Geometry: final body of the model. Coordinates: model frame, mm. Face numbers are marked on the shaded views. A direction names the side the tool comes from. Give positions to 0.01 mm unless a question says otherwise; leave off trailing zeros. Order: outer loops, then holes, each group sorted by start corner. A loop starts at its lowest first (then second) coordinate and runs counter-clockwise, first axis right, second up. Notation, with made-up numbers: (-37, 82) -> (-26, 82) arc R17 ccw to (-26, 96) -> close; hole circle Ø4 at (76, 22). An arc over 180 degrees is marked (long way). One line per item, written item: value. Start each with the question number.
```python
from build123d import *

# Parameters (mm, degrees)
BOSS_EXTRUDE1_DEPTH     = 7.5
CUT_EXTRUDE1_REACH      = 84.651
SKETCH2_R               = 5
CUT_EXTRUDE2_REACH      = 89.839
CUT_EXTRUDE2_END_RADIUS = 39.885527085
SKETCH3_R               = 5


with BuildPart() as part:
    # Sketch1 → Boss-Extrude1 (new, symmetric)
    with BuildSketch(Plane(origin=(0, 0, 0), x_dir=(1, 0, 0), z_dir=(0, 1, 0))):
        with BuildLine():
            Line((-17.171350292, -36), (17.171350292, -36))
            ThreePointArc((17.171350292, -36), (39.885527085, 0), (17.171350292, 36))
            Line((17.171350292, 36), (-17.171350292, 36))
            ThreePointArc((-17.171350292, 36), (-39.885527085, 0), (-17.171350292, -36))
        make_face()
        with BuildLine():
            Line((-16, 31), (16, 31))
            ThreePointArc((16, 31), (34.885527085, 0), (16, -31))
            Line((16, -31), (-16, -31))
            ThreePointArc((-16, -31), (-34.885527085, 0), (-16, 31))
        make_face(mode=Mode.SUBTRACT)
    extrude(amount=BOSS_EXTRUDE1_DEPTH, both=True)

    # Cut-Extrude1: up to this face of the body (flat: up to its plane)
    cut_extrude1_end = Plane(part.part.faces().sort_by_distance((0, 0, -36))[0])
    # Sketch2 → Cut-Extrude1 (cut, up to the picked face)
    with BuildSketch(Plane.XY.offset(36), mode=Mode.PRIVATE) as cut_extrude1_sk1:
        with Locations((0, -0.5)):
            Circle(SKETCH2_R)
    cut_extrude1_tool1 = split(extrude(cut_extrude1_sk1.sketch, amount=-CUT_EXTRUDE1_REACH, mode=Mode.PRIVATE), bisect_by=cut_extrude1_end, keep=Keep.BOTH, mode=Mode.PRIVATE)
    add(cut_extrude1_tool1.solids().sort_by(Axis((0, -0.5, 36), (0, 0, -1)))[0], mode=Mode.SUBTRACT)

    # Cut-Extrude2: up to this cylinder (the profile starts inside it)
    cut_extrude2_end = Plane(origin=(0, 0, 0), z_dir=(0, -1, 0)) * Cylinder(CUT_EXTRUDE2_END_RADIUS, 260.44905417, mode=Mode.PRIVATE)
    # Sketch3 → Cut-Extrude2 (cut, up to the surface)
    with BuildSketch(Plane.ZY.offset(39.885527085), mode=Mode.PRIVATE) as cut_extrude2_sk1:
        Circle(SKETCH3_R)
    cut_extrude2_tool1 = extrude(cut_extrude2_sk1.sketch, amount=-CUT_EXTRUDE2_REACH, mode=Mode.PRIVATE) & cut_extrude2_end
    add(cut_extrude2_tool1.solids().sort_by_distance((-39.885527, 0, 0))[0], mode=Mode.SUBTRACT)


solid = part.part
```
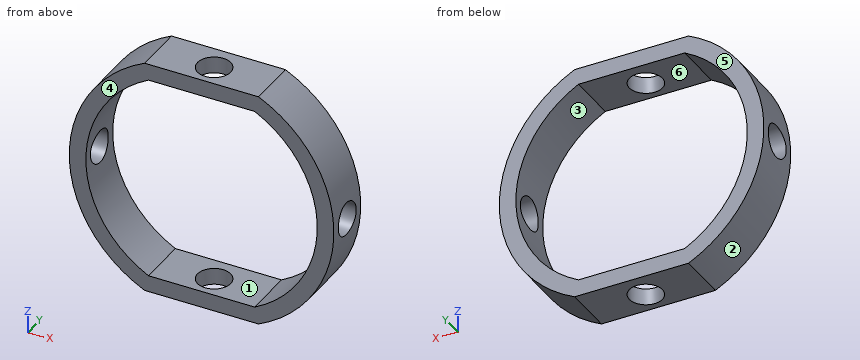
1. Cut plane C-C, the plane y = 1. Return loops of the section in (x, z), then the cut area to 3 significant figures.
2. Pin query (flat end, axial travel): P1, Ø5, axis at x = -22, y = 4, coming from the -Z side; P2, Ø8, axis at y = -6, z = -13, coming from the -X side; P3, Ø6, axis at y = 5, z = 23, coming from the -X side. Return the tip coordinate at first contact, or that it passes through.
3. Cut plane A-A, the plane z = 0. Return loops of the section in (x, y), then the cut area to 3 significant figures.
4. Material intervals for L1, parallel to Z at x = 5.5, y = 1.5; L2, parallel to Y at x = 0, z = -33.7; L3, parallel to Y at x = 37.9, z = 0, sorted ascending. Write a range as [from, to].
5. Access query for the marked faces 5 and 6. Directions: +Z, -Z, +X, -X, +Y, -Y. A direction counts if a zero-diameter tool reaches every point of the face in a straight line with its end or side. Return the directions, or none.
6. Draft query along X for the marked faces 1, 2, 3 and 4. Return one class per face: pulls with the +X half, pulls with the -X half, needs draft (parallel to the pull), parting line crosses it, or undercut.
7. Cut plane D-D, the plane x = -26.5. Return loops of the section in (y, z).
8. Cut plane B-B, the plane x = 0. Return loops of the section in (y, z), then the cut area to 3 significant figures.
Answers follow:
1. outline: (-39.58, -4.9) arc R39.89 ccw to (-17.17, -36) -> (-4.77, -36) -> (-4.77, -31) -> (-16, -31) arc R34.89 cw to (-34.54, -4.9) -> close; (-39.58, 4.9) -> (-34.54, 4.9) arc R34.89 cw to (-16, 31) -> (-4.77, 31) -> (-4.77, 36) -> (-17.17, 36) arc R39.89 ccw to start; (4.77, -36) -> (17.17, -36) arc R39.89 ccw to (39.58, -4.9) -> (34.54, -4.9) arc R34.89 cw to (16, -31) -> (4.77, -31) -> close; (4.77, 31) -> (16, 31) arc R34.89 cw to (34.54, 4.9) -> (39.58, 4.9) arc R39.89 ccw to (17.17, 36) -> (4.77, 36) -> close
1. area: 969 mm²
2. P1: stops at z = -34.79
2. P2: stops at x = -38.86
2. P3: stops at x = -34.51
3. outline: (-39.89, -7.5) -> (-34.89, -7.5) -> (-34.89, -5) -> (-39.89, -5) -> close; (-39.89, 5) -> (-34.89, 5) -> (-34.89, 7.5) -> (-39.89, 7.5) -> close; (34.89, -7.5) -> (39.89, -7.5) -> (39.89, -5) -> (34.89, -5) -> close; (34.89, 5) -> (39.89, 5) -> (39.89, 7.5) -> (34.89, 7.5) -> close
3. area: 50.0 mm²
4. L1: z = [-36, -31], [31, 36]
4. L2: y = [-7.5, -5.5], [4.5, 7.5]
4. L3: y = [-7.5, -5], [5, 7.5]
5. face 5: +Z, -Z, +X, -X, +Y
5. face 6: +Y, -Y
6. face 1: undercut
6. face 2: pulls with the -X half
6. face 3: undercut
6. face 4: needs draft
7. outline: (-7.5, -29.81) -> (7.5, -29.81) -> (7.5, -22.69) -> (-7.5, -22.69) -> close; (-7.5, 22.69) -> (7.5, 22.69) -> (7.5, 29.81) -> (-7.5, 29.81) -> close
8. outline: (-7.5, -36) -> (-5.5, -36) -> (-5.5, -31) -> (-7.5, -31) -> close; (-7.5, 31) -> (-5.5, 31) -> (-5.5, 36) -> (-7.5, 36) -> close; (4.5, -36) -> (7.5, -36) -> (7.5, -31) -> (4.5, -31) -> close; (4.5, 31) -> (7.5, 31) -> (7.5, 36) -> (4.5, 36) -> close
8. area: 50.0 mm²
